```python
from build123d import *

# Parameters (mm, degrees)
BOSS_EXTRUDE1_DEPTH = 2.3
SKETCH7_W           = 2.3
SKETCH7_H           = 10
SKETCH7_W_2         = 10
SKETCH7_H_2         = 2.3
CUT_EXTRUDE2_DEPTH  = 3.3
SKETCH9_R           = 1
CUT_EXTRUDE4_DEPTH  = 3.3
SKETCH10_W          = 3
SKETCH10_H          = 15
SKETCH10_W_2        = 25
SKETCH10_H_2        = 7.5
CUT_EXTRUDE5_DEPTH  = 3.3
FILLET2_R           = 1
FILLET3_R           = 2
SKETCH11_R          = 3
CUT_EXTRUDE6_DEPTH  = 10


with BuildPart() as part:
    # Sketch1 → Boss-Extrude1 (new body)
    with BuildSketch(Plane.XY):
        Polygon((0, -57), (0, -90), (23, -90), (77, -90), (100, -90), (100, -57), (100, 0), (0, 0), align=None)
    extrude(amount=BOSS_EXTRUDE1_DEPTH)

    # Sketch7 → Cut-Extrude2 (cut, through all)
    with BuildSketch(Plane.XY.offset(2.3)):
        with Locations((91, -15)):
            Rectangle(SKETCH7_W, SKETCH7_H)
        with Locations((91, -45)):
            Rectangle(SKETCH7_W, SKETCH7_H)
        with Locations((9, -15)):
            Rectangle(SKETCH7_W, SKETCH7_H)
        with Locations((9, -45)):
            Rectangle(SKETCH7_W, SKETCH7_H)
        with Locations((37.5, -86)):
            Rectangle(SKETCH7_W_2, SKETCH7_H_2)
        with Locations((62.5, -86)):
            Rectangle(SKETCH7_W_2, SKETCH7_H_2)
    extrude(amount=-CUT_EXTRUDE2_DEPTH, mode=Mode.SUBTRACT)

    # Sketch9 → Cut-Extrude4 (cut, through all)
    with BuildSketch(Plane.XY.offset(2.3)):
        with Locations((3, -3)):
            Circle(SKETCH9_R)
        with Locations((97, -3)):
            Circle(SKETCH9_R)
        with Locations((41.13, -11.4)):
            Circle(SKETCH9_R)
        with Locations((69.03, -11.4)):
            Circle(SKETCH9_R)
        with Locations((25.89, -62.2)):
            Circle(SKETCH9_R)
        with Locations((74.11, -63.5)):
            Circle(SKETCH9_R)
    extrude(amount=-CUT_EXTRUDE4_DEPTH, mode=Mode.SUBTRACT)

    # Sketch10 → Cut-Extrude5 (cut, through all)
    with BuildSketch(Plane.XY.offset(2.3)):
        with Locations((17, -22.5)):
            Rectangle(SKETCH10_W, SKETCH10_H)
        with Locations((83, -22.5)):
            Rectangle(SKETCH10_W, SKETCH10_H)
        with Locations((50, -78.75)):
            Rectangle(SKETCH10_W_2, SKETCH10_H_2)
    extrude(amount=-CUT_EXTRUDE5_DEPTH, mode=Mode.SUBTRACT)

    # Fillet2
    fillet2_edges = [part.edges().sort_by_distance(p)[0] for p in [
        (15.5, -30, 1.15),
        (15.5, -15, 1.15),
        (18.5, -15, 1.15),
        (18.5, -30, 1.15),
        (81.5, -30, 1.15),
        (81.5, -15, 1.15),
        (84.5, -15, 1.15),
        (84.5, -30, 1.15),
    ]]
    fillet(fillet2_edges, radius=FILLET2_R)

    # Fillet3
    fillet3_edges = [part.edges().sort_by_distance(p)[0] for p in [
        (37.5, -82.5, 1.15),
        (37.5, -75, 1.15),
        (62.5, -75, 1.15),
        (62.5, -82.5, 1.15),
    ]]
    fillet(fillet3_edges, radius=FILLET3_R)

    # Sketch11 → Cut-Extrude6 (cut)
    with BuildSketch(Plane.XY.offset(2.3)):
        with Locations((94, -58)):
            Circle(SKETCH11_R)
    extrude(amount=-CUT_EXTRUDE6_DEPTH, mode=Mode.SUBTRACT)


solid = part.part
```
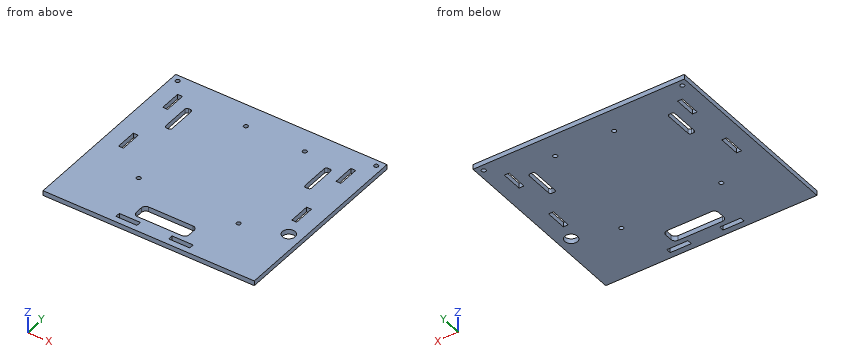
Input: part model. Units: mm. Frame: model coordinates. Give positions to 0.01 mm unless a question says otherwise; leave off trailing zeros. Order: outer loops, then holes, each group sorted by start corner. A loop starts at its lowest first (then second) coordinate and runs counter-clockwise, first axis right, second up. Notation, with made-up numbers: M 13,68 L 54,68 A12 ccw 54,91 Z; hole C -29,22 d3. An arc over 180 degrees is marked long. Return JSON: item names as keys, results as strings.
1) Section query C-C on y = -79. Output: boundary loops of the cut face in (x, z), and give its area (4 significant figures).
Taken from the geometry:
{"outline": "M 0,0 L 37.5,0 L 37.5,2.3 L 0,2.3 Z; M 62.5,0 L 100,0 L 100,2.3 L 62.5,2.3 Z", "area": "172.5 mm2"}
2) Section query B-B on y = -45. Output: boundary loops of the cut face in (x, z).
Taken from the geometry:
{"outline": "M 0,0 L 7.85,0 L 7.85,2.3 L 0,2.3 Z; M 10.15,0 L 89.85,0 L 89.85,2.3 L 10.15,2.3 Z; M 92.15,0 L 100,0 L 100,2.3 L 92.15,2.3 Z"}
3) Line query: L1, parallel to Y at x = 8, z = 2.2; L2, parallel to Y at x = 59.5, z = 0.5; L3, parallel to X at y = -28, z = 0.7. Output: solid intervals per line, ascending. Write a range as [from, to].
Taken from the geometry:
{"L1": "y = [-90, -50], [-40, -20], [-10, 0]", "L2": "y = [-90, -87.15], [-84.85, -82.5], [-75, 0]", "L3": "x = [0, 15.5], [18.5, 81.5], [84.5, 100]"}
4) Section query A-A on x = 94. Output: boundary loops of the cut face in (y, z).
Taken from the geometry:
{"outline": "M -90,0 L -61,0 L -61,2.3 L -90,2.3 Z; M -55,0 L 0,0 L 0,2.3 L -55,2.3 Z"}
5) Section query D-D on z = 0.9. Count the separate pieces of the cut face and the enclosed holes in it, and give its area (3 significant figures).
Taken from the geometry:
{"separate pieces": "1", "enclosed holes": "16", "area": "8,540 mm2"}
